from build123d import *

# Parameters (mm, degrees)
F0_W     = 6.25
F0_H     = 24.75
F0_R     = 2.25
F1_ANGLE = 30
F2_DEPTH = 12.5
F0_H_2   = 24
F0_R_2   = 2
F3_ANGLE = 15
F4_DEPTH = 5


with BuildPart() as f1:
    # F0 (on Right) → F1 (revolve, symmetric)
    with BuildSketch(Plane.YZ) as f1_sk:
        with Locations((-22.875, 48.987537)):
            Rectangle(F0_W, F0_H)
        with Locations((-22.875, 40.737537)):
            Circle(F0_R, mode=Mode.SUBTRACT)
        with Locations((-22.875, 48.987537)):
            Circle(F0_R, mode=Mode.SUBTRACT)
        with Locations((-22.875, 57.237537)):
            Circle(F0_R, mode=Mode.SUBTRACT)
        with Locations((-22.875, 57.237537)):
            Circle(F0_R)
        with Locations((-22.875, 48.987537)):
            Circle(F0_R)
        with Locations((-22.875, 40.737537)):
            Circle(F0_R)
    revolve(axis=Axis((0, 0, 63), (0, 0, 1)), revolution_arc=F1_ANGLE / 2)
    revolve(f1_sk.sketch, axis=Axis((0, 0, 63), (0, 0, -1)), revolution_arc=F1_ANGLE / 2)

    # F0 (on Right) → F2 (cut, symmetric)
    with BuildSketch(Plane.YZ):
        with Locations((-22.875, 57.237537)):
            Circle(F0_R)
        with Locations((-22.875, 48.987537)):
            Circle(F0_R)
        with Locations((-22.875, 40.737537)):
            Circle(F0_R)
    extrude(amount=F2_DEPTH, both=True, mode=Mode.SUBTRACT)

    # F0 (on Right) → F3 (revolve, symmetric)
    with BuildSketch(Plane.YZ) as f3_sk:
        with Locations((-22.875, 24.612537)):
            Rectangle(F0_W, F0_H_2)
        with Locations((-22.875, 15.612537)):
            Circle(F0_R_2, mode=Mode.SUBTRACT)
        with Locations((-22.875, 21.612537)):
            Circle(F0_R_2, mode=Mode.SUBTRACT)
        with Locations((-22.875, 27.612537)):
            Circle(F0_R_2, mode=Mode.SUBTRACT)
        with Locations((-22.875, 33.612537)):
            Circle(F0_R_2, mode=Mode.SUBTRACT)
        with Locations((-22.875, 33.612537)):
            Circle(F0_R_2)
        with Locations((-22.875, 27.612537)):
            Circle(F0_R_2)
        with Locations((-22.875, 21.612537)):
            Circle(F0_R_2)
        with Locations((-22.875, 15.612537)):
            Circle(F0_R_2)
    revolve(axis=Axis((0, 0, 63), (0, 0, 1)), revolution_arc=F3_ANGLE / 2)
    revolve(f3_sk.sketch, axis=Axis((0, 0, 63), (0, 0, -1)), revolution_arc=F3_ANGLE / 2)

    # F0 (on Right) → F4 (cut, symmetric)
    with BuildSketch(Plane.YZ):
        with Locations((-22.875, 33.612537)):
            Circle(F0_R_2)
        with Locations((-22.875, 27.612537)):
            Circle(F0_R_2)
        with Locations((-22.875, 21.612537)):
            Circle(F0_R_2)
        with Locations((-22.875, 15.612537)):
            Circle(F0_R_2)
    extrude(amount=F4_DEPTH, both=True, mode=Mode.SUBTRACT)


solid = f1.part
Geometry: final body of the model. Coordinates: model frame, mm. A direction names the side the tool comes from. Give positions to 0.01 mm unless a question says otherwise; leave off trailing zeros. Write each loop counter-clockwise with the first axis right and the second up, starting at its lowest first coordinate (ties: lowest second). Pieces come first, ordered by that corner, then holes. Notation, with made-up numbers: (75, -20.75) - (127, -20.75) arc R35 cw to (127, 11.25) - close; hole circle Ø6 at (36, 61.5). An arc over 180 degrees is marked (long way). Return JSON: item names as keys, results as strings. Group by question number.
1) Section A-A on x = 1. Return the cut outline in (y, z) (3 decimals).
2) Set-up query: faces 4 (the flat face through (0, -23, 12.613)), 5 (the flat face through (-2.99, -22.72, 24.78)), 6 (the flat face through (2.99, -22.72, 24.78)). Return all of +Z, -Z, +X, -X, +Y, -Y with unobstructed straight access to the full face (end or side cutting, diameter ignored); none if empty.
3) Section B-B on z = 56. Return the cut outline in (x, y), plus the area to 3 significant figures.
4) Section D-D on z = 18.5. Return the cut outline in (x, y).
5) Line query: line 1 (Z direction, x = -5.5, y = -21.75); line 2 (Z direction, x = -3.5, y = -19.5); line 3 (Z direction, x = -3, y = -21.5). Output: solid intervals per line, ascending.
6) First-contact query: P1, Ø6, axis at x = -2, z = 46.5, coming from the +Y side; P2, Ø2, axis at x = 5.5, y = -22, coming from the -Z side; P3, Ø3, axis at y = -24, z = 30.5, coming from the -X side; P4, Ø3, axis at x = -1, z = 49.5, coming from the -Y side. Flat tips, straight axial feed; report the tip coordinate or a pass-through.
7) Section C-C on y = -23.5. State how many separate pieces and enclosed holes the cut face has, plus the area to 3 significant figures.
8) Mould query, pull axis Y, two halves, no side actions, for faces 1 (the cylindrical face through (0, -26, 43)), 2 (the flat face through (-5, -22, 36.613)), 3 (the cylindrical face through (0.046, -24.873, 21.7)). Classes: released by +Y, released by -Y, zero draft, split by the parting line, or undercut.
Filled in:
{
 "1": {"outline": "(-25.981, 12.613) - (-19.725, 12.613) - (-19.725, 61.363) - (-25.981, 61.363) - close; hole circle Ø4.5 at (-22.875, 40.738); hole circle Ø4.5 at (-22.875, 48.988); hole circle Ø4.5 at (-22.875, 57.238); hole circle Ø4 at (-22.875, 15.613); hole circle Ø4 at (-22.875, 21.613); hole circle Ø4 at (-22.875, 27.613); hole circle Ø4 at (-22.875, 33.613)"},
 "2": {"face 4": "-Z, +X, -X, +Y, -Y", "face 5": "-Z, -X, +Y", "face 6": "-Z, +X, +Y"},
 "3": {"outline": "(-6.73, -25.11) arc R26 ccw to (6.73, -25.11) - (6.63, -24.75) - (-6.63, -24.75) - close; (-5.63, -21) - (5.63, -21) - (5.11, -19.08) arc R19.75 cw to (-5.11, -19.08) - close", "area": "28.8 mm^2"},
 "4": {"outline": "(-3.39, -25.78) arc R26 ccw to (3.39, -25.78) - (2.58, -19.58) arc R19.75 cw to (-2.58, -19.58) - close"},
 "5": {"line 1": "z = 36.61 to 38.79, 42.69 to 47.04, 50.94 to 55.29, 59.19 to 61.36", "line 2": "z = 36.61 to 61.36", "line 3": "z = 36.61 to 38.96, 42.52 to 47.21, 50.77 to 55.46, 59.02 to 61.36"},
 "6": {"P1": "stops at y = -19.11", "P2": "stops at z = 36.61", "P3": "stops at x = -3.36", "P4": "stops at y = -26"},
 "7": {"separate pieces": "8", "enclosed holes": "0", "area": "203 mm^2"},
 "8": {"face 1": "released by -Y", "face 2": "zero draft", "face 3": "undercut"}
}
